The listing builds one solid part. Answer for the finished solid, in the listing's coordinates (mm). A direction names the side the tool comes from. Give positions to 0.01 mm unless a question says otherwise; leave off trailing zeros. Loops run counter-clockwise (first coordinate to the right, second up) from the corner with the lowest first, then second, coordinate; pieces in that order, holes last.
Item 1: Section A-A, the plane x = 0 is taken. Give the vertices of the cut face in (y, z).
Item 2: The mould has two halves that part along Y. Classify faces 1 (the face through (9.63, -7.57, 38.54)), 2 (the face through (3.35, -6.43, 71.49)), 3 (the face through (-11, -7, 5.5)): pulls with the +Y half, pulls with the -Y half, needs draft (parallel to the pull), parting line crosses it, or undercut.
Item 3: Each of these flat-tipped pins is pushed along its axis until it touches: pin 1 Ø3 at (x, z) = (12, 63.5) entering from -Y; pin 2 Ø6 at (x, z) = (-9.5, 46.5) entering from +Y; pin 3 Ø6 at (x, z) = (5.5, 27.5) entering from +Y. Where does it stop, or does it pass through?
Item 4: Consider line 1 along Y through (x, z) = (0, 33.5); line 2 along Y through (x, z) = (0, 71.7). Determine where each line is inside the solid, lowest interval first.
Item 5: Section C-C, the plane z = 26 is taken. Give the vertices of the cut face in (x, y).
Item 6: A tool of negligible diameter and unlimited length cuts with its end or side. For faces 4 (the face through (11, -3, 0)), 5 (the face through (-2.778, 8.823, 35.524)), from which of +Z, -Z, +X, -X, +Y, -Y can it reach the whole face along a straight path? Write none if from no direction.
from build123d import *

# Parameters (mm, degrees)
SKETCH1_R           = 12.25
SKETCH1_R_2         = 9.25
EXTRUDE_THIN1_DEPTH = 70
SKETCH3_R           = 15.75
SKETCH3_R_2         = 10.75
EXTRUDE_THIN2_DEPTH = 5.5
SKETCH4_R           = 12.25
SKETCH4_R_2         = 7.25
EXTRUDE_THIN3_DEPTH = 2


with BuildPart() as part:
    # Sketch1 → Extrude-Thin1 (new body)
    with BuildSketch(Plane(origin=(0, 0, 0), x_dir=(0, 1, 0), z_dir=(0, 0, 1))):
        Circle(SKETCH1_R)
        Circle(SKETCH1_R_2, mode=Mode.SUBTRACT)
    extrude(amount=EXTRUDE_THIN1_DEPTH)

    # Sketch3 → Extrude-Thin2 (add)
    with BuildSketch(Plane(origin=(0, 0, 0), x_dir=(0, 1, 0), z_dir=(0, 0, 1))):
        Circle(SKETCH3_R)
        Circle(SKETCH3_R_2, mode=Mode.SUBTRACT)
    extrude(amount=EXTRUDE_THIN2_DEPTH)

    # Sketch4 → Extrude-Thin3 (add)
    with BuildSketch(Plane.XY.offset(70)):
        Circle(SKETCH4_R)
        Circle(SKETCH4_R_2, mode=Mode.SUBTRACT)
    extrude(amount=EXTRUDE_THIN3_DEPTH)

    # Chamfer1: read off the stored shape, not the designer's step
    # Chamfer1 outline → Chamfer1 (revolve, cut)
    with BuildSketch(Plane.XZ):
        Polygon((9.25, 2), (9.25, 0), (11.25, 0), align=None)
        Polygon((15.75, 1), (14.75, 0), (15.75, 0), align=None)
        Polygon((7.25, 70), (8.25, 70), (7.25, 71), align=None)
        Polygon((14.75, 5.5), (15.75, 4.5), (15.75, 5.5), align=None)
    revolve(axis=Axis((0, 0, 0), (0, 0, 1)), mode=Mode.SUBTRACT)

    # Chamfer1 2 outline → Chamfer1 2 (revolve)
    with BuildSketch(Plane.XZ):
        Polygon((12.25, 6), (12.25, 5.5), (12.75, 5.5), align=None)
    revolve(axis=Axis((0, 0, 0), (0, 0, 1)))


solid = part.part
Worked answers:
1. outline: (-15.75, 1) - (-14.75, 0) - (-11.25, 0) - (-9.25, 2) - (-9.25, 70) - (-8.25, 70) - (-7.25, 71) - (-7.25, 72) - (-12.25, 72) - (-12.25, 6) - (-12.75, 5.5) - (-14.75, 5.5) - (-15.75, 4.5) - close; (7.25, 71) - (8.25, 70) - (9.25, 70) - (9.25, 2) - (11.25, 0) - (14.75, 0) - (15.75, 1) - (15.75, 4.5) - (14.75, 5.5) - (12.75, 5.5) - (12.25, 6) - (12.25, 72) - (7.25, 72) - close
2. face 1: parting line crosses it
2. face 2: undercut
2. face 3: needs draft
3. pin 1: stops at y = -6.31
3. pin 2: stops at y = 10.38
3. pin 3: stops at y = 11.99
4. line 1: y = -12.25 to -9.25, 9.25 to 12.25
4. line 2: y = -12.25 to -7.25, 7.25 to 12.25
5. outline: circle Ø24.5 at (0, 0); hole circle Ø18.5 at (0, 0)
6. face 4: -Z, +X, -X, +Y, -Y
6. face 5: -Z
